The listing builds one solid part. Answer for the finished solid, in the listing's coordinates (mm). A direction names the side the tool comes from. Coordinates: 2 decimals unless noted, no trailing zeros. Answer as CSV lines item,"result".
```python
from build123d import *

# Parameters (mm, degrees)
CYLINDER001_R     = 6
CYLINDER001_DEPTH = 10
CYLINDER_R        = 6
CYLINDER_DEPTH    = 10
EXTRUDE_DEPTH     = 10


with BuildPart() as cilindro001:
    # Cylinder001 → Cylinder001 (new body)
    with BuildSketch(Plane(origin=(54, -39, 8), x_dir=(1, 0, 0), z_dir=(0, 0, 1))):
        Circle(CYLINDER001_R)
    extrude(amount=CYLINDER001_DEPTH)


with BuildPart() as fusion:
    # Cylinder → Cylinder (new body)
    with BuildSketch(Plane(origin=(30, -39, 8), x_dir=(1, 0, 0), z_dir=(0, 0, 1))):
        Circle(CYLINDER_R)
    extrude(amount=CYLINDER_DEPTH)

    # Fusion: union Cilindro001
    add(cilindro001.part)


with BuildPart() as cut:
    # path4136 → Extrude (new body)
    with BuildSketch(Plane(origin=(42.376579, -44.354878, 0), x_dir=(0, -1, 0), z_dir=(0, 0, -1))):
        with BuildLine():
            add(Edge.make_bspline(
                [(-13.85455, 35.407203), (-13.85455, 35.407203), (-37.333463, 51.129846), (-42.46778, 34.856929)],
                knots=[0, 0, 0, 0, 1, 1, 1, 1], degree=3))
            add(Edge.make_bspline(
                [(-42.46778, 34.856929), (-47.602099, 18.584013), (-19.100017, 16.70568), (-19.100017, 16.70568)],
                knots=[0, 0, 0, 0, 1, 1, 1, 1], degree=3))
            add(Edge.make_bspline(
                [(-19.100017, 16.70568), (-19.100017, 16.70568), (-25.576689, 12.757134), (-25.65703, -0.546311)],
                knots=[0, 0, 0, 0, 1, 1, 1, 1], degree=3))
            add(Edge.make_bspline(
                [(-25.65703, -0.546311), (-25.73737, -13.849756), (-18.52984, -19.647173), (-18.52984, -19.647173)],
                knots=[0, 0, 0, 0, 1, 1, 1, 1], degree=3))
            add(Edge.make_bspline(
                [(-18.52984, -19.647173), (-18.52984, -19.647173), (-45.927429, -13.606641), (-44.129391, -32.51663)],
                knots=[0, 0, 0, 0, 1, 1, 1, 1], degree=3))
            add(Edge.make_bspline(
                [(-44.129391, -32.51663), (-42.331353, -51.426623), (-12.828091, -34.756809), (-12.828091, -34.756809)],
                knots=[0, 0, 0, 0, 1, 1, 1, 1], degree=3))
            add(Edge.make_bspline(
                [(-12.828091, -34.756809), (-12.828091, -34.756809), (44.732088, -31.969997), (45.329759, -0.261224)],
                knots=[0, 0, 0, 0, 1, 1, 1, 1], degree=3))
            add(Edge.make_bspline(
                [(45.329759, -0.261224), (45.927429, 31.447549), (-13.85455, 35.407203), (-13.85455, 35.407203)],
                knots=[0, 0, 0, 0, 1, 1, 1, 1], degree=3))
        make_face()
    extrude(amount=-EXTRUDE_DEPTH)

    # Cut: cut Fusion
    add(fusion.part, mode=Mode.SUBTRACT)


with BuildPart() as cut_1:
    # Cut placement: moved
    add(cut.part.moved(Location((-42, 0, 0))))


solid = cut_1.part
```
Q1. Straight lines are drawn through the part: line 1 (X direction, y = -39, z = 8.65); line 2 (X direction, y = -22, z = 6.75); line 3 (Y direction, x = -12, z = 9.55). For each, find the intervals that lie inside material, in ascending order.
Output:
line 1,"-34.04 to -18, -6 to 6, 18 to 34.41"
line 2,"-39.49 to -16.7, -12.68 to 15.05, 19.42 to 39.45"
line 3,"-86.18 to -45, -33 to -21.6"
Q2. The mould has two halves that part along Y. Classify faces 1 (the flat face through (0, -43, 0)), 2 (the flat face through (-12, -39, 8)): pulls with the +Y half, pulls with the -Y half, needs draft (parallel to the pull), parting line crosses it, or undercut.
Output:
face 1,"needs draft"
face 2,"undercut"
Q3. Flat-ended cylindrical pins translate along their axes: pin 1 Ø10 at (x, y) = (25, -58.5) entering from -Z; pin 2 Ø6 at (x, y) = (11.5, -40) entering from +Z; pin 3 Ø1 at (x, z) = (-25, 5) entering from -Y; pin 4 Ø3 at (x, z) = (25, 4.5) entering from -Y. Find the tip coordinate at first contact, or state that the pin passes through.
Output:
pin 1,"z = 0"
pin 2,"z = 8"
pin 3,"y = -71.38"
pin 4,"y = -74.63"
Q4. For faces 3 (the cylindrical face through (-9.231, -44.323, 8.986)), 4 (the flat face through (0, -43, 10)), determine the directions among +Z, -Z, +X, -X, +Y, -Y from which every point of the face is accessible in a straight line to the end or side of a thin tool.
Output:
face 3,"+Z"
face 4,"+Z, +X, -X, +Y, -Y"
